Can you work these out from the model? Positions are in its coordinate system, mm. Face numbers are marked on the shaded views. A direction names the side the tool comes from. Give positions to 0.01 mm unless a question says otherwise; leave off trailing zeros. Order: outer loops, then holes, each group sorted by start corner. A loop starts at its lowest first (then second) coordinate and runs counter-clockwise, first axis right, second up. Notation, with made-up numbers: (-25.5, 0.25) - (18.5, 0.25) arc R28 ccw to (18.5, 38.25) - close; hole circle Ø11 at (79.25, 75.5). An arc over 180 degrees is marked (long way). Use one line per item in the form item = value. Start each with the question number.
1) For pin 1 (5 mm diameter, centred on x = 2, y = 150.5, fed in from -Z); pin 2 (5 mm diameter, centred on x = 3, y = 175, fed in from +Z); pin 3 (5 mm diameter, centred on x = -1, y = 155, fed in from +Z), each with a flat end and sliding along its axis, tell me the tip position at first contact or that it passes through.
2) We'd pull the mould along Y, two halves only. Please class the marked faces 4, 5 and 6: released by +Y, released by -Y, zero draft, split by the parting line, or undercut.
3) Suppose I cut it at B-B, the plane x = -1.5. Write out the boundary of the cut face in (y, z).
4) Suppose I cut it at D-D, the plane x = 1. Write out the boundary of the cut face in (y, z), and give its area (3 significant figures).
5) Suppose I cut it at C-C, the plane z = -109.5. Write out the boundary of the cut face in (x, y), and give its area (3 significant figures).
6) Which directions (+Z, -Z, +X, -X, +Y, -Y) give clear straight access to the entire face, cutting with the end or side of a thin tool? Please do the marked faces 1, 2 and 3.
7) Please list where these lines run through material, in increasing order: probe 1 along Y at (x, z) = (0.5, -120.5); probe 2 along Z at (x, y) = (0, 169.5); probe 3 along Y at (x, z) = (3.25, -123).
8) Suppose I cut it at A-A, the plane z = -114. Write out the boundary of the cut face in (x, y).
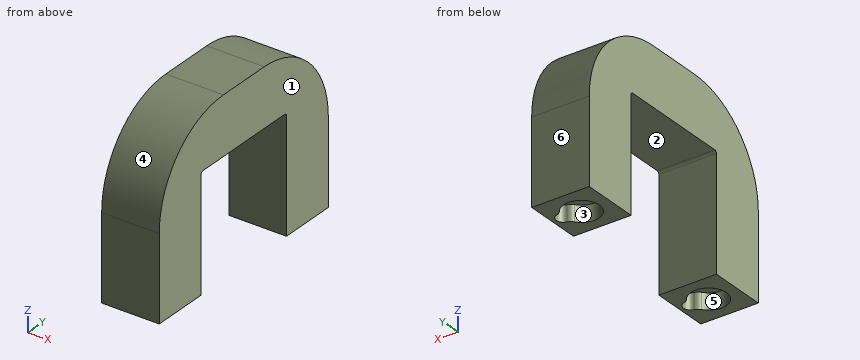
```python
from build123d import *

# Parameters (mm, degrees)
SALIENTE_EXTRUIR1_DEPTH = 10
CROQUIS3_R              = 3.1
CROQUIS3_R_2            = 1.25
CORTAR_EXTRUIR1_DEPTH   = 4
REDONDEO2_R             = 1.5


with BuildPart() as part:
    # Croquis2 → Saliente-Extruir1 (new body)
    with BuildSketch(Plane(origin=(-2.525360123, 2.123276243, -2.466894012), x_dir=(0, 0, -1), z_dir=(1, 0, 0))):
        with BuildLine():
            Line((103.598862982, 173.647805519), (108.516020269, 173.647805519))
            Line((108.516020269, 173.647805519), (118.281705694, 173.647805519))
            Line((118.281705694, 173.647805519), (123.198862982, 173.647805519))
            Line((123.198862982, 173.647805519), (123.198862982, 183.647805519))
            Line((123.198862982, 183.647805519), (118.281705694, 183.647805519))
            Line((118.281705694, 183.647805519), (108.516020269, 183.647805519))
            ThreePointArc((108.516020269, 183.647805519), (97.685154483, 179.161514018), (93.198862982, 168.330648231))
            Line((93.198862982, 168.330648231), (93.198862982, 158.564962806))
            ThreePointArc((93.198862982, 158.564962806), (97.685154483, 147.73409702), (108.516020269, 143.247805519))
            Line((108.516020269, 143.247805519), (118.281705694, 143.247805519))
            Line((118.281705694, 143.247805519), (123.198862982, 143.247805519))
            Line((123.198862982, 143.247805519), (123.198862982, 153.247805519))
            Line((123.198862982, 153.247805519), (118.281705694, 153.247805519))
            Line((118.281705694, 153.247805519), (108.516020269, 153.247805519))
            Line((108.516020269, 153.247805519), (103.598862982, 153.247805519))
            ThreePointArc((103.598862982, 153.247805519), (103.316020269, 153.364962806), (103.198862982, 153.647805519))
            Line((103.198862982, 153.647805519), (103.198862982, 158.564962806))
            Line((103.198862982, 158.564962806), (103.198862982, 168.330648231))
            Line((103.198862982, 168.330648231), (103.198862982, 173.247805519))
            ThreePointArc((103.198862982, 173.247805519), (103.316020269, 173.530648231), (103.598862982, 173.647805519))
        make_face()
    extrude(amount=SALIENTE_EXTRUIR1_DEPTH)

    # Croquis3 → Cortar-Extruir1 (cut)
    with BuildSketch(Plane(origin=(0, 0, -126.865756994), x_dir=(-1, 0, 0), z_dir=(0, 0, -1))):
        with Locations((-2.474639877, 150.371081761)):
            Circle(CROQUIS3_R)
        with Locations((-2.474639877, 180.771081761)):
            Circle(CROQUIS3_R)
        with Locations((-5.574639877, 180.771081761)):
            Circle(CROQUIS3_R_2)
        with Locations((-5.574639877, 150.371081761)):
            Circle(CROQUIS3_R_2)
    extrude(amount=-CORTAR_EXTRUIR1_DEPTH, mode=Mode.SUBTRACT)

    # Redondeo2
    redondeo2_edges = [part.edges().sort_by_distance(p)[0] for p in [
        (5.322623748, 179.54675016, -124.265756994),
        (5.322623748, 181.995413363, -124.265756994),
        (5.322623748, 151.595413363, -124.265756994),
        (5.322623748, 149.14675016, -124.265756994),
    ]]
    fillet(redondeo2_edges, radius=REDONDEO2_R)


solid = part.part
```
Result sheet:
q1.pin_1 = -122.87
q1.pin_2 = -95.8
q1.pin_3 = -96
q2.face_4 = released by -Y
q2.face_5 = undercut
q2.face_6 = released by +Y
q3.outline = (145.37, -125.67) - (155.37, -125.67) - (155.37, -106.07) arc R0.4 cw to (155.77, -105.67) - (175.37, -105.67) arc R0.4 cw to (175.77, -106.07) - (175.77, -125.67) - (185.77, -125.67) - (185.77, -110.98) arc R15.32 ccw to (170.45, -95.67) - (160.69, -95.67) arc R15.32 ccw to (145.37, -110.98) - close
q4.outline = (145.37, -125.67) - (147.64, -125.67) - (147.64, -122.87) - (153.1, -122.87) - (153.1, -125.67) - (155.37, -125.67) - (155.37, -106.07) arc R0.4 cw to (155.77, -105.67) - (175.37, -105.67) arc R0.4 cw to (175.77, -106.07) - (175.77, -125.67) - (178.04, -125.67) - (178.04, -122.87) - (183.5, -122.87) - (183.5, -125.67) - (185.77, -125.67) - (185.77, -110.98) arc R15.32 ccw to (170.45, -95.67) - (160.69, -95.67) arc R15.32 ccw to (145.37, -110.98) - close
q4.area = 673 mm²
q5.outline = (-2.53, 145.44) - (7.47, 145.44) - (7.47, 155.37) - (-2.53, 155.37) - close; (-2.53, 175.77) - (7.47, 175.77) - (7.47, 185.7) - (-2.53, 185.7) - close
q5.area = 199 mm²
q6.face_1 = +Z, -Z, +X, +Y, -Y
q6.face_2 = -Z, +X, -X
q6.face_3 = -Z
q7.probe_1 = 145.37 to 155.37, 175.77 to 185.77
q7.probe_2 = -105.67 to -95.67
q7.probe_3 = 145.37 to 147.37, 153.37 to 155.37, 175.77 to 177.77, 183.77 to 185.77
q8.outline = (-2.53, 145.37) - (7.47, 145.37) - (7.47, 155.37) - (-2.53, 155.37) - close; (-2.53, 175.77) - (7.47, 175.77) - (7.47, 185.77) - (-2.53, 185.77) - close
